from build123d import *

# Parameters (mm, degrees)
EXTRUDE_1_DEPTH = 5


with BuildPart() as part:
    # 草图1 → 凸台-拉伸1 (new body)
    with BuildSketch(Plane(origin=(0, 0, 0), x_dir=(1, 0, 0), z_dir=(0, 1, 0))):
        Polygon((30, -20.08), (30, 0), (0, 0), (0, -60), (30, -60), (30, -52.18), (24.1, -52.18), (24.1, -48.18), (24.1, -24.38), (24.1, -20.08), align=None)
        Polygon((60, 0), (30, 0), (30, -20.08), (35.9, -20.08), (35.9, -24.38), (35.9, -48.18), (35.9, -52.18), (30, -52.18), (30, -60), (60, -60), align=None)
        with BuildLine():
            Line((30, -48.18), (24.1, -48.18))
            Line((24.1, -48.18), (24.1, -52.18))
            Line((24.1, -52.18), (30, -52.18))
            Line((30, -52.18), (30, -51.23))
            ThreePointArc((30, -51.23), (28.9, -50.13), (30, -49.03))
            Line((30, -49.03), (30, -48.18))
        make_face()
        with BuildLine():
            Line((35.9, -52.18), (35.9, -48.18))
            Line((35.9, -48.18), (30, -48.18))
            Line((30, -48.18), (30, -49.03))
            ThreePointArc((30, -49.03), (30.777817459, -49.352182541), (31.1, -50.13))
            ThreePointArc((31.1, -50.13), (30.777817459, -50.907817459), (30, -51.23))
            Line((30, -51.23), (30, -52.18))
            Line((30, -52.18), (35.9, -52.18))
        make_face()
        with BuildLine():
            Line((30, -21.03), (30, -20.08))
            Line((30, -20.08), (24.1, -20.08))
            Line((24.1, -20.08), (24.1, -24.38))
            Line((24.1, -24.38), (30, -24.38))
            Line((30, -24.38), (30, -23.23))
            ThreePointArc((30, -23.23), (28.9, -22.13), (30, -21.03))
        make_face()
        with BuildLine():
            Line((35.9, -20.08), (30, -20.08))
            Line((30, -20.08), (30, -21.03))
            ThreePointArc((30, -21.03), (30.777817459, -21.352182541), (31.1, -22.13))
            ThreePointArc((31.1, -22.13), (30.777817459, -22.907817459), (30, -23.23))
            Line((30, -23.23), (30, -24.38))
            Line((30, -24.38), (35.9, -24.38))
            Line((35.9, -24.38), (35.9, -20.08))
        make_face()
    extrude(amount=EXTRUDE_1_DEPTH)


solid = part.part
Part model, mm, in its own coordinate system. A direction names the side the tool comes from. Coordinates: 2 decimals unless noted, no trailing zeros. Write each loop counter-clockwise with the first axis right and the second up, starting at its lowest first coordinate (ties: lowest second). Pieces come first, ordered by that corner, then holes. Notation, with made-up numbers: (83.5, -4.75) - (90.5, -4.75) arc R18 cw to (90.5, 10.25) - close; hole circle Ø1 at (16, -27.5). An arc over 180 degrees is marked (long way). Put each result on its own line as item: value.
1. Band-saw the part on A-A (y = 2). Write the cut outline in (x, z), then the cut area to 3 significant figures.
Final values:
outline: (0, 0) - (60, 0) - (60, 60) - (0, 60) - close; hole (24.1, 24.38) - (35.9, 24.38) - (35.9, 48.18) - (24.1, 48.18) - close; hole circle Ø2.2 at (30, 22.13); hole circle Ø2.2 at (30, 50.13)
area: 3,310 mm²
2. Probe line 1 along X through (y, z) = (3.85, 50); line 2 along Z through (x, y) = (27, 1.65); line 3 along X through (y, z) = (1.35, 29.5). List the from-to ranges inside material, lowest first. Write a range as [from, to].
Final values:
line 1: x = [0, 28.91], [31.09, 60]
line 2: z = [0, 24.38], [48.18, 60]
line 3: x = [0, 24.1], [35.9, 60]
3. Band-saw the part on B-B (z = 41.5). Write the cut outline in (x, y), then the cut area to 3 significant figures.
Final values:
outline: (0, 0) - (24.1, 0) - (24.1, 5) - (0, 5) - close; (35.9, 0) - (60, 0) - (60, 5) - (35.9, 5) - close
area: 241 mm²
4. Two-plate mould, pull along Z, no slides. Class faces 3 (the flat face through (30, 2, 0)), 4 (the flat face through (30, 2, 60)), 5 (the flat face through (24.1, 2, 36)), 6 (the flat face through (23, 5, 30)): +Z half, -Z half, draft (parallel to the pull), parting line (faces both ways), or undercut.
Final values:
face 3: -Z half
face 4: +Z half
face 5: undercut
face 6: draft
5. 3-axis set-ups, long thin cutter, end or side, ignore diameter. For faces 1 (the flat face through (30, 2, 48.18)), 2 (the flat face through (60, 2, 30)): which of +Z, -Z, +X, -X, +Y, -Y reach the whole face in a straight line?
Final values:
face 1: +Y, -Y
face 2: +Z, -Z, +X, +Y, -Y
